from build123d import *

# Parameters (mm, degrees)
BOSS_EXTRUDE1_DEPTH  = 3.5
SKETCH2_W            = 4
SKETCH2_H            = 10
CUT_EXTRUDE1_DEPTH   = 2.5
FILLET1_R            = 1
FILLET2_R            = 1
FILLET2_OF_MIRROR1_R = 1
SKETCH3_W            = 9
SKETCH3_H            = 8.290227197
CUT_EXTRUDE3_DEPTH   = 2
CHAMFER2_START       = 4.709772803
CHAMFER2_DEPTH       = 8.290227197
CHAMFER2_START_2     = 3
CHAMFER2_2_DEPTH     = 2.09807924
CHAMFER3_SIZE        = 1
M3_CLEARANCE_HOLE2_D = 3.6
FILLET4_R            = 2
SKETCH13_W           = 12.5
SKETCH13_H           = 6
CUT_EXTRUDE4_DEPTH   = 2
CHAMFER4_SIZE        = 2


with BuildPart() as part:
    # Sketch1 → Boss-Extrude1 (new body)
    with BuildSketch(Plane(origin=(0, 0, 0), x_dir=(1, 0, 0), z_dir=(0, 1, 0))):
        Polygon((-4.5, -6.25), (-15, -6.25), (-15, 6.25), (15, 6.25), (15, -6.25), (4.5, -6.25), (4.5, -13), (-4.5, -13), align=None)
    extrude(amount=BOSS_EXTRUDE1_DEPTH)

    # Sketch2 → Cut-Extrude1 (cut)
    with BuildSketch(Plane.XZ):
        with Locations((-11, 0)):
            Rectangle(SKETCH2_W, SKETCH2_H)
    cut_extrude1 = extrude(amount=-CUT_EXTRUDE1_DEPTH, mode=Mode.SUBTRACT)

    # Fillet1
    fillet1_edges = [part.edges().sort_by_distance(p)[0] for p in [
        (-15, 1.75, -6.25),
        (15, 1.75, -6.25),
        (15, 1.75, 6.25),
        (4.5, 1.75, 6.25),
        (-4.5, 1.75, 6.25),
        (-15, 1.75, 6.25),
    ]]
    fillet(fillet1_edges, radius=FILLET1_R)

    # Fillet2
    fillet2_edges = [part.edges().sort_by_distance(p)[0] for p in [
        (-9, 1.25, 5),
        (-9, 1.25, -5),
        (-13, 1.25, -5),
        (-13, 1.25, 5),
    ]]
    fillet(fillet2_edges, radius=FILLET2_R)

    # Mirror1: Cut-Extrude1 across plane
    add(cut_extrude1.mirror(Plane(origin=(0, 0, 0), x_dir=(0, 0, 1), z_dir=(1, 0, 0))), mode=Mode.SUBTRACT)

    # Fillet2 of Mirror1
    fillet2_of_mirror1_edges = [part.edges().sort_by_distance(p)[0] for p in [
        (9, 1.25, 5),
        (9, 1.25, -5),
        (13, 1.25, -5),
        (13, 1.25, 5),
    ]]
    fillet(fillet2_of_mirror1_edges, radius=FILLET2_OF_MIRROR1_R)

    # Sketch3 → Cut-Extrude3 (cut)
    with BuildSketch(Plane(origin=(0, 3.5, 0), x_dir=(1, 0, 0), z_dir=(0, 1, 0))):
        with Locations((0, -8.854886401)):
            Rectangle(SKETCH3_W, SKETCH3_H)
    extrude(amount=-CUT_EXTRUDE3_DEPTH, mode=Mode.SUBTRACT)

    # Chamfer2: read off the stored shape, not the designer's step
    # Chamfer2 outline → Chamfer2 (add)
    with BuildSketch(Plane.XY.offset(CHAMFER2_START)):
        Polygon((4.5, 2.5), (3.5, 1.5), (4.5, 1.5), align=None)
        Polygon((-4.5, 2.5), (-4.5, 1.5), (-3.5, 1.5), align=None)
    extrude(amount=CHAMFER2_DEPTH)

    # Chamfer2 2 outline → Chamfer2 2 (add)
    with BuildSketch(Plane(origin=(0, 0, 0), x_dir=(1, 0, 0), z_dir=(0, 0.70710678118655, 0.707106781186545)).offset(CHAMFER2_START_2)):
        Polygon((4.5, -1.562545334), (-4.5, -1.562545334), (-3.5, -2.976758896), (3.5, -2.976758896), align=None)
    extrude(amount=CHAMFER2_2_DEPTH)

    # Chamfer3
    chamfer3_edges = [part.edges().sort_by_distance(p)[0] for p in [
        (-4.792893219, 3.5, 6.542893219),
        (-9.75, 3.5, 6.25),
        (-14.707106781, 3.5, 5.957106781),
        (-15, 3.5, 0),
        (-14.707106781, 3.5, -5.957106781),
        (0, 3.5, -6.25),
        (14.707106781, 3.5, -5.957106781),
        (15, 3.5, 0),
        (14.707106781, 3.5, 5.957106781),
        (9.75, 3.5, 6.25),
        (4.792893219, 3.5, 6.542893219),
        (4.5, 3.5, 5.979886401),
        (0, 3.5, 4.709772803),
        (-4.5, 3.5, 5.979886401),
    ]]
    chamfer(chamfer3_edges, length=CHAMFER3_SIZE - 0.0001)  # a hair under: the kernel refuses the full size

    # M3 Clearance Hole2 (through all)
    with Locations(Plane(origin=(0, 1.5, 0), x_dir=(1, 0, 0), z_dir=(0, 1, 0))):
        with Locations((0, -9.75)):
            Hole(M3_CLEARANCE_HOLE2_D / 2)

    # Fillet4
    fillet4_edges = [part.edges().sort_by_distance(p)[0] for p in [
        (4.5, 1.25, 13),
        (-4.5, 1.25, 13),
    ]]
    fillet(fillet4_edges, radius=FILLET4_R)

    # Sketch13 → Cut-Extrude4 (cut)
    with BuildSketch(Plane(origin=(0, 3.5, 0), x_dir=(1, 0, 0), z_dir=(0, 1, 0))):
        with Locations((0, 0.75)):
            Rectangle(SKETCH13_W, SKETCH13_H)
    extrude(amount=-CUT_EXTRUDE4_DEPTH, mode=Mode.SUBTRACT)

    # Chamfer4
    chamfer4_edges = [part.edges().sort_by_distance(p)[0] for p in [
        (0, 1.5, -3.75),
        (6.25, 1.5, -0.75),
        (0, 1.5, 2.25),
        (-6.25, 1.5, -0.75),
    ]]
    chamfer(chamfer4_edges, length=CHAMFER4_SIZE - 0.0001)  # a hair under: the kernel refuses the full size


solid = part.part
Input: part model. Units: mm. Frame: model coordinates. A direction names the side the tool comes from. Give positions to 0.01 mm unless a question says otherwise; leave off trailing zeros. Write each loop counter-clockwise with the first axis right and the second up, starting at its lowest first coordinate (ties: lowest second). Pieces come first, ordered by that corner, then holes. Notation, with made-up numbers: (-5.75, 16.25) -> (-0.75, 16.25) arc R29 ccw to (-0.75, 43.25) -> close; hole circle Ø1 at (88, -38). An arc over 180 degrees is marked (long way). Use one line per item in the form item = value. Start each with the question number.
1) Pin query (flat end, axial travel): pin 1 (2 mm diameter, centred on x = 11.5, z = 2, fed in from -Y); pin 2 (1 mm diameter, centred on x = 1.5, y = 2.5, fed in from +Z); pin 3 (0.6 mm diameter, centred on x = -11, y = 1.5, fed in from +Z). Return the tip coordinate at first contact, or that it passes through.
2) Ray query, probe 1 along X at (y, z) = (0.85, 2.25); probe 2 along Z at (x, y) = (-10.75, 2.1); probe 3 along Z at (x, y) = (0, 0.45). Return the intervals inside material, ascending. Write a range as from..to.
3) Section query B-B on y = 0.6. Count the separate pieces of the cut face and the enclosed holes in it, then the cut area to 3 significant figures.
4) Section query C-C on z = 9.75. Return the cut outline in (x, y).
5) Draft query along X for faces 1 (the flat face through (-10, 1, 6.25)), 2 (the flat face through (9, 1, 0)), 3 (the flat face through (-15, 1, 0)). Return one class per face: pulls with the +X half, pulls with the -X half, needs draft (parallel to the pull), parting line crosses it, or undercut.
6) Set-up query: faces 4 (the flat face through (-0.06, 2.01, 5.2)), 5 (the flat face through (-0.09, 2.49, 1.24)), 6 (the cylindrical face through (9.301, 1.268, 4.715)), 7 (the flat face through (-4.5, 1, 9)). Return all of +Z, -Z, +X, -X, +Y, -Y with unobstructed straight access to the full face (end or side cutting, diameter ignored); none if empty.
7) Section query D-D on x = 7. Return the cut outline in (y, z).
Outcome:
q1.pin_1 = 2.5
q1.pin_2 = 5.21
q1.pin_3 = 6.25
q2.probe_1 = -15..-13, -9..9, 13..15
q2.probe_2 = -6.25..-5, 5..6.25
q2.probe_3 = -6.25..7.95, 11.55..13
q3.separate_pieces = 1
q3.enclosed_holes = 3
q3.area = 345 mm^2
q4.outline = (-4.5, 0) -> (-1.8, 0) -> (-1.8, 1.5) -> (-3.5, 1.5) -> (-4.5, 2.5) -> close; (1.8, 0) -> (4.5, 0) -> (4.5, 2.5) -> (3.5, 1.5) -> (1.8, 1.5) -> close
q5.face_1 = needs draft
q5.face_2 = undercut
q5.face_3 = pulls with the -X half
q6.face_4 = +Z, +Y
q6.face_5 = +Y
q6.face_6 = -Y
q6.face_7 = +Z, -X, +Y, -Y
q7.outline = (0, -6.25) -> (2.5, -6.25) -> (3.5, -5.25) -> (3.5, 5.25) -> (2.5, 6.25) -> (0, 6.25) -> close
